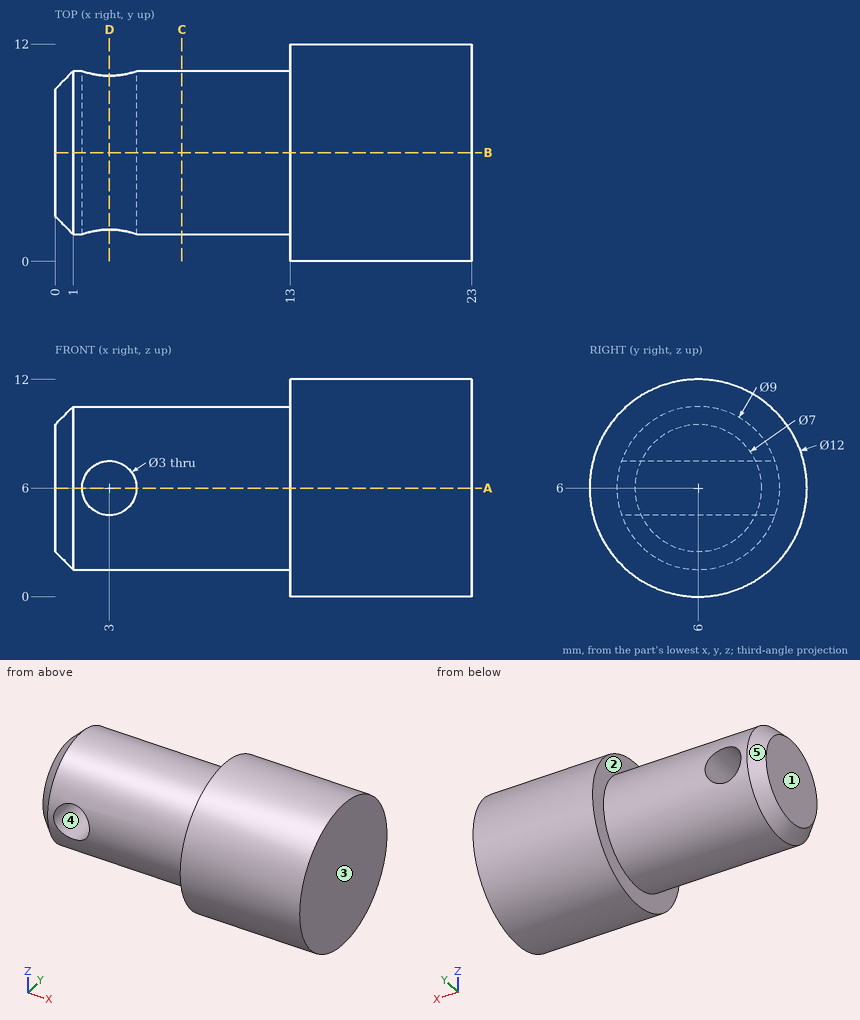
Input: dimensioned drawing with shaded views. Units: mm. Origin: part minimum x, y, z. A direction names the side the tool comes from. Round coordinates to 2 decimals unless told otherwise and drop trailing zeros. Write each loop counter-clockwise with the first axis right and the second up, starting at its lowest first coordinate (ties: lowest second). Pieces come first, ordered by that corner, then holes. Notation, with made-up numbers: (53, -34.75) - (86, -34.75) arc R18 cw to (86, -25.75) - close; hole circle Ø10 at (81, 78). An arc over 180 degrees is marked (long way). Write item = value, one per line.
(1) Section query B-B on y = 6. Output: boundary loops of the cut face in (x, z).
Geometry check:
outline = (0, 2.5) - (1, 1.5) - (13, 1.5) - (13, 0) - (23, 0) - (23, 12) - (13, 12) - (13, 10.5) - (1, 10.5) - (0, 9.5) - close; hole circle Ø3 at (3, 6)
(2) Section query D-D on x = 3. Output: boundary loops of the cut face in (y, z).
Geometry check:
outline = (1.76, 4.5) arc R4.5 ccw to (10.24, 4.5) - close; (1.76, 7.5) - (10.24, 7.5) arc R4.5 ccw to start
(3) Section query C-C on x = 7. Output: boundary loops of the cut face in (y, z), then the cut area to 3 significant figures.
Geometry check:
outline = circle Ø9 at (6, 6)
area = 63.6 mm^2
(4) Access query for the marked faces 1 and 2. Directions: +Z, -Z, +X, -X, +Y, -Y. A direction counts if a zero-diameter tool reaches every point of the face in a straight line with its end or side. Return the directions, or none.
Geometry check:
face_1 = +Z, -Z, -X, +Y, -Y
face_2 = -X
(5) Material intervals for probe 1 along X at (y, z) = (7, 6); probe 2 along Z at (x, y) = (3, 7); probe 3 along Y at (x, z) = (14.75, 6.25), sorted ascending.
Geometry check:
probe_1 = 0 to 1.5, 4.5 to 23
probe_2 = 1.61 to 4.5, 7.5 to 10.39
probe_3 = 0.01 to 11.99
(6) Section query A-A on z = 6. Output: boundary loops of the cut face in (x, y), then the cut area to 3 significant figures.
Geometry check:
outline = (0, 2.5) - (1, 1.5) - (1.5, 1.5) - (1.5, 10.5) - (1, 10.5) - (0, 9.5) - close; (4.5, 1.5) - (13, 1.5) - (13, 0) - (23, 0) - (23, 12) - (13, 12) - (13, 10.5) - (4.5, 10.5) - close
area = 209 mm^2
(7) Contact query for flat-ended pins moving along their axis: pin 1 Ø2.5 at (x, z) = (3, 6) entering from -Y; pin 2 Ø2 at (x, z) = (7, 4.5) entering from +Y; pin 3 Ø6 at (x, z) = (9.5, 8.5) entering from -Y; pin 4 Ø2 at (x, z) = (4, 1.5) entering from -Y. Output: stop coordinate, or through.
Geometry check:
pin_1 = through
pin_2 = 10.47
pin_3 = 1.5
pin_4 = 3.17
(8) Pull-direction query (Z, two-part tool) for the marked faces 3, 4 and 5; classes: +Z half, -Z half, draft (parallel to the pull), parting line (faces both ways), or undercut.
Geometry check:
face_3 = draft
face_4 = undercut
face_5 = parting line
